Design review of the part built by this model. Coordinates are the model's own, in mm. A direction names the side the tool comes from. Give positions to 0.01 mm unless a question says otherwise; leave off trailing zeros. Loops run counter-clockwise (first coordinate to the right, second up) from the corner with the lowest first, then second, coordinate; pieces in that order, holes last. Notation, with made-up numbers: M -17,-29 L -6,-29 A9 cw -6,-21 Z; hole C -29.75,67 d11. An arc over 180 degrees is marked long. Use a Markdown table: item, result. Add a question column.
(1) Add section B-B, the plane x = 5. Give the boundary of the cut face in (y, z).
(2) Draft analysis for pull direction Z (two halves, no side actions). For faces 1 (the face through (5, 5, 20)), 2 (the face through (4.62, 14.4, 43.29)), 3 (the face through (5, 30, 25)), state which applies: pulls with the +Z half, pulls with the -Z half, needs draft (parallel to the pull), parting line crosses it, or undercut.
(3) For faces 4 (the face through (5, 25, 20)), 5 (the face through (5, 19, 50)), 6 (the face through (5, 4, 25)), 7 (the face through (5, 22, 45)), list the 3-axis set-ups (+Z, -Z, +X, -X, +Y, -Y) from which the entire face can be reached by the end or side of a thin tool; tool diameter is ignored.
(4) Insertion check: pin 1 Ø4 at (x, z) = (5, 45) entering from -Y; pin 2 Ø1.8 at (x, z) = (5.5, 45) entering from -Y; pin 3 Ø2 at (x, y) = (5, 5) entering from +Z. Each pin has a flat end and moves straight along its axis. Give the tip position at first contact, or say it passes through.
(5) Add section D-D, the plane z = 14. Give the boundary of the cut face in (x, y).
(6) For probe 1 along Y at (x, z) = (5, 5.5); probe 2 along Z at (x, y) = (5, 10.5); probe 3 along Y at (x, z) = (3.5, 7), list the stretches that pass through material, from the lowest coordinate up.
(7) Add section A-A, the plane z = 45. Give the boundary of the cut face in (x, y), then the cut area to 4 significant figures.
(8) Add section C-C, the plane y = 15. Give the boundary of the cut face in (x, z), then the cut area to 3 significant figures.
```python
from build123d import *

# Parameters (mm, degrees)
ESQUISSE1_W             = 10
ESQUISSE1_H             = 30
ESQUISSE1_R             = 1.75
BOSS_EXTRU_1_DEPTH      = 20
ESQUISSE2_W             = 10
ESQUISSE2_H             = 30
BOSS_EXTRU_2_DEPTH      = 5
ESQUISSE3_W             = 10
ESQUISSE3_H             = 23
BOSS_EXTRU_3_DEPTH      = 25
ESQUISSE4_R             = 1.75
ENL_V_MAT_EXTRU_1_DEPTH = 15


with BuildPart() as part:
    # Esquisse1 → Boss.-Extru.1 (new body)
    with BuildSketch(Plane.XY):
        with Locations((5, 15)):
            Rectangle(ESQUISSE1_W, ESQUISSE1_H)
        with Locations((5, 5)):
            Circle(ESQUISSE1_R, mode=Mode.SUBTRACT)
        with Locations((5, 15)):
            Circle(ESQUISSE1_R, mode=Mode.SUBTRACT)
        with Locations((5, 25)):
            Circle(ESQUISSE1_R, mode=Mode.SUBTRACT)
    extrude(amount=BOSS_EXTRU_1_DEPTH)

    # Esquisse2 → Boss.-Extru.2 (add)
    with BuildSketch(Plane.XY.offset(20)):
        with Locations((5, 15)):
            Rectangle(ESQUISSE2_W, ESQUISSE2_H)
    extrude(amount=BOSS_EXTRU_2_DEPTH)

    # Esquisse3 → Boss.-Extru.3 (add)
    with BuildSketch(Plane.XY.offset(25)):
        with Locations((5, 18.5)):
            Rectangle(ESQUISSE3_W, ESQUISSE3_H)
    extrude(amount=BOSS_EXTRU_3_DEPTH)

    # Esquisse4 → Enlèv. mat.-Extru.1 (cut)
    with BuildSketch(Plane(origin=(0, 7, 0), x_dir=(-1, 0, 0), z_dir=(0, -1, 0))):
        with Locations(Location((-5, -45, 0), (0, 0, 180))):
            Circle(ESQUISSE4_R)
        with Locations(Location((-5, -35, 0), (0, 0, 180))):
            Circle(ESQUISSE4_R)
    extrude(amount=-ENL_V_MAT_EXTRU_1_DEPTH, mode=Mode.SUBTRACT)


solid = part.part
```
Established:
| question | item | result |
|---|---|---|
| 1 | outline | M 0,0 L 3.25,0 L 3.25,20 L 6.75,20 L 6.75,0 L 13.25,0 L 13.25,20 L 16.75,20 L 16.75,0 L 23.25,0 L 23.25,20 L 26.75,20 L 26.75,0 L 30,0 L 30,50 L 7,50 L 7,46.75 L 22,46.75 L 22,43.25 L 7,43.25 L 7,36.75 L 22,36.75 L 22,33.25 L 7,33.25 L 7,25 L 0,25 Z |
| 2 | face 1 | pulls with the -Z half |
| 2 | face 2 | undercut |
| 2 | face 3 | needs draft |
| 3 | face 4 | -Z |
| 3 | face 5 | +Z, +X, -X, +Y, -Y |
| 3 | face 6 | +Z, +X, -X, -Y |
| 3 | face 7 | -Y |
| 4 | pin 1 | y = 7 |
| 4 | pin 2 | y = 22 |
| 4 | pin 3 | z = 25 |
| 5 | outline | M 0,0 L 10,0 L 10,30 L 0,30 Z; hole C 5,5 d3.5; hole C 5,15 d3.5; hole C 5,25 d3.5 |
| 6 | probe 1 | 0 to 3.25, 6.75 to 13.25, 16.75 to 23.25, 26.75 to 30 |
| 6 | probe 2 | 0 to 33.25, 36.75 to 43.25, 46.75 to 50 |
| 6 | probe 3 | 0 to 4.1, 5.9 to 14.1, 15.9 to 24.1, 25.9 to 30 |
| 7 | outline | M 0,7 L 3.25,7 L 3.25,22 L 6.75,22 L 6.75,7 L 10,7 L 10,30 L 0,30 Z |
| 7 | area | 177.5 mm^2 |
| 8 | outline | M 0,0 L 3.25,0 L 3.25,20 L 6.75,20 L 6.75,0 L 10,0 L 10,50 L 0,50 Z; hole C 5,35 d3.5; hole C 5,45 d3.5 |
| 8 | area | 411 mm^2 |
